Can you work these out from the model? Positions are in its coordinate system, mm. Give positions to 0.01 mm unless a question says otherwise; leave off trailing zeros.
from build123d import *

# Parameters (mm, degrees)
SKETCH1_W                  = 650
SKETCH1_H                  = 300
BOSS_EXTRUDE1_DEPTH        = 20
FILLET1_R                  = 10
F_11_0_11_DIAMETER_HOLE1_D = 11
F_7_0_7_DIAMETER_HOLE2_D   = 7
F_4_0_4_DIAMETER_HOLE1_D   = 4
M8_CLEARANCE_HOLE1_D       = 8.4


with BuildPart() as part:
    # Sketch1 → Boss-Extrude1 (new body)
    with BuildSketch(Plane(origin=(0, 0, 0), x_dir=(0, 0, -1), z_dir=(1, 0, 0))):
        with Locations((325, 150)):
            Rectangle(SKETCH1_W, SKETCH1_H)
    extrude(amount=BOSS_EXTRUDE1_DEPTH)

    # Fillet1
    fillet1_edges = [part.edges().sort_by_distance(p)[0] for p in [
        (10, 300, 0),
        (10, 300, -650),
        (10, 0, -650),
        (10, 0, 0),
    ]]
    fillet(fillet1_edges, radius=FILLET1_R)

    # Ø11.0 (11) Diameter Hole1 (through all)
    with Locations(Plane(origin=(20, 0, 0), x_dir=(0, 0, -1), z_dir=(1, 0, 0))):
        with Locations((54.646833709, 244.998152891), (530.659083677, 81.560470498), (510.229373378, 207.543684009), (244.64313949, 63.173731229), (181.992027906, 188.475954397), (351.558623389, 207.543684009), (370.626353001, 71.345615349), (76.438524695, 125.143852469), (450.302223168, 145.573562769), (450.302223168, 263.38489216)):
            Hole(F_11_0_11_DIAMETER_HOLE1_D / 2)

    # Ø7.0 (7) Diameter Hole2 (through all)
    with Locations(Plane(origin=(20, 0, 0), x_dir=(0, 0, -1), z_dir=(1, 0, 0))):
        with Locations((107.764080486, 44.106001616), (224.213429191, 129.910784873), (246.005120177, 239.550230144), (487.075701706, 95.861267707), (382.203188837, 151.021485515), (577.647417365, 249.765085294), (602.844060068, 55.001847109)):
            Hole(F_7_0_7_DIAMETER_HOLE2_D / 2)

    # Ø4.0 (4) Diameter Hole1 (through all)
    with Locations(Plane(origin=(20, 0, 0), x_dir=(0, 0, -1), z_dir=(1, 0, 0))):
        with Locations((152.709443144, 251.12706598), (88.696350874, 186.432983367), (297.760386268, 170.089215127), (346.791690986, 265.42786319), (535.426016081, 150.340495172), (442.811329391, 41.382040243)):
            Hole(F_4_0_4_DIAMETER_HOLE1_D / 2)

    # M8 Clearance Hole1 (through all)
    with Locations(Plane.ZY):
        with Locations((-625, 235.86), (-625, 70), (-25, 70), (-25, 235.86)):
            Hole(M8_CLEARANCE_HOLE1_D / 2)


solid = part.part
(1) Will this pin go through, and if not, where does the flat tip stop? P1, Ø17.5, axis at y = 263.38, z = -450.3, coming from the +X side.
Returned:
P1: stops at x = 20
(2) Thinking about a two-plate mould opening in Z: for faces 1 (the flat face through (10, 0, -321)), 2 (the cylindrical face through (9.86, 81.802, -536.154)), 3 (the flat face through (10, 148, -650)), which applies, pulls with the +Z half, pulls with the -Z half, needs draft (parallel to the pull), parting line crosses it, or undercut?
Returned:
face 1: needs draft
face 2: undercut
face 3: pulls with the -Z half
(3) Please list where these lines run through material, in increasing order: probe 1 along Z at (x, y) = (3.5, 211); probe 2 along Z at (x, y) = (4.25, 212.5); probe 3 along Z at (x, y) = (2.75, 237.5).
Returned:
probe 1: z = -650 to -514.51, -505.95 to -355.84, -347.28 to 0
probe 2: z = -650 to -512.61, -507.85 to -353.94, -349.17 to 0
probe 3: z = -650 to -628.87, -621.13 to -248.84, -243.17 to -28.87, -21.13 to 0
